Verification items for the finished model (mm, model axes). Face numbers are marked on the shaded views. A direction names the side the tool comes from. Coordinates: 2 decimals unless noted, no trailing zeros. Write each loop counter-clockwise with the first axis right and the second up, starting at its lowest first coordinate (ties: lowest second). Pieces come first, ordered by that corner, then holes. Notation, with made-up numbers: (33.25, -27) -> (70.25, -27) arc R27 ccw to (70.25, -8) -> close; hole circle Ø7 at (14, -19.5). An arc over 180 degrees is marked (long way). Use a Markdown table: item, result. Add a question column.
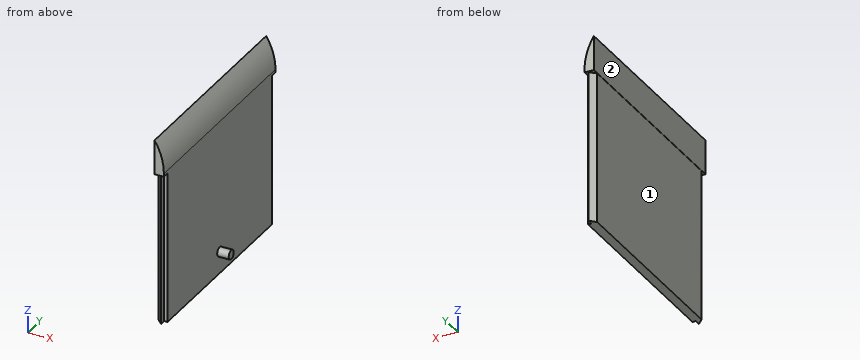
from build123d import *

# Parameters (mm, degrees)
BOSS_EXTRUDE1_DEPTH = 105
BOSS_EXTRUDE2_DEPTH = 24
FILLET1_R           = 40
SKETCH5_R           = 3.219097994
BOSS_EXTRUDE3_DEPTH = 8


with BuildPart() as part:
    # Sketch1 → Boss-Extrude1 (new body)
    with BuildSketch(Plane.XY):
        Polygon((37.684072543, -12), (37.684072543, -7.95), (33.684072543, -12), (33.684072543, -148), (37.684072543, -152.05), (37.684072543, -148), (40, -148), (40, -12), align=None)
    extrude(amount=-BOSS_EXTRUDE1_DEPTH)

    # Sketch4 → Boss-Extrude2 (add)
    with BuildSketch(Plane.XY):
        Polygon((40, -152.75), (33.5, -152.75), (33.5, -7.25), (40, -7.25), (40, -80), align=None)
    extrude(amount=BOSS_EXTRUDE2_DEPTH)

    # Fillet1
    # the kernel refuses this fillet: 40 mm, written as the material it takes off along each edge
    with BuildSketch(Plane(origin=(40, 47.393732486, 24), x_dir=(0, 0, -1), z_dir=(0, -1, 0))) as fillet1_piece_1:
        with BuildLine():
            CenterArc((21.857492994, -40), FILLET1_R, 90, 33.122940208)
            Line((0, -6.5), (-0.43714986, -5.83))
            ThreePointArc((-0.43714986, -5.83), (-0.8, -3.25), (-0.8, 0))
            Line((-0.8, 0), (0, 0.8))
            Line((0, 0.8), (21.857492994, 0.8))
            Line((21.857492994, 0.8), (21.857492994, 0))
        make_face()
    extrude(amount=254.787464972, mode=Mode.SUBTRACT)

    # Sketch5 → Boss-Extrude3 (add)
    with BuildSketch(Plane(origin=(40, 0, 0), x_dir=(0, 0, -1), z_dir=(1, 0, 0))):
        with Locations((89.714756259, -80)):
            Circle(SKETCH5_R)
    extrude(amount=BOSS_EXTRUDE3_DEPTH)


solid = part.part
1) Gauge pin test, flat ends, axial feed: pin 1 (1.5 mm diameter, centred on x = 42, z = -34.5, fed in from -Y); pin 2 (0.7 mm diameter, centred on x = 38.5, z = -42.5, fed in from +Y); pin 3 (2 mm diameter, centred on y = -120.5, z = -28, fed in from -X); pin 4 (0.7 mm diameter, centred on x = 39.5, z = -77.5, fed in from -Y). Record the tip position at first contact, or that the pin passes through.
2) Cross-section at C-C on x = 45.75. Record the boundary of the cut face in (y, z), then the cut area to 3 significant figures.
3) Cross-section at B-B on y = -80. Record the boundary of the cut face in (x, z).
4) Cross-section at D-D on z = 16. Record the boundary of the cut face in (x, y), then the cut area to 3 significant figures.
5) Set-up check for the marked faces 1 and 2: record each of +Z, -Z, +X, -X, +Y, -Y from which the full face is reachable in a straight line by a thin tool's end or side.
6) Cross-section at A-A on z = -7. Record the boundary of the cut face in (x, y), then the cut area to 3 significant figures.
7) Thickness scan on L1, parallel to Y at x = 39, z = -15; L2, parallel to X at y = -124, z = -10.5; L3, parallel to Z at x = 36, y = -18. Record the ranges inside material, lowest first.
Returned:
| question | item | result |
|---|---|---|
| 1 | pin 1 | passes through |
| 1 | pin 2 | stops at y = -12 |
| 1 | pin 3 | stops at x = 33.68 |
| 1 | pin 4 | stops at y = -148 |
| 2 | outline | circle Ø6.44 at (-80, -89.71) |
| 2 | area | 32.6 mm² |
| 3 | outline | (33.5, 0) -> (33.68, 0) -> (33.68, -105) -> (40, -105) -> (40, -92.93) -> (48, -92.93) -> (48, -86.5) -> (40, -86.5) -> (40, 2.14) arc R40 ccw to (33.5, 24) -> close |
| 4 | outline | (33.5, -152.75) -> (37.52, -152.75) -> (37.52, -7.25) -> (33.5, -7.25) -> close |
| 4 | area | 585 mm² |
| 5 | face 1 | -Z, -X, +Y, -Y |
| 5 | face 2 | +Z, -Z, -X, +Y, -Y |
| 6 | outline | (33.68, -148) -> (37.68, -152.05) -> (37.68, -148) -> (40, -148) -> (40, -12) -> (37.68, -12) -> (37.68, -7.95) -> (33.68, -12) -> close |
| 6 | area | 875 mm² |
| 7 | L1 | y = -148 to -12 |
| 7 | L2 | x = 33.68 to 40 |
| 7 | L3 | z = -105 to 19.58 |
